Work out the finished part from the listing and answer in its coordinate system (mm). Face numbers are marked on the shaded views. A direction names the side the tool comes from. Coordinates: 2 decimals unless noted, no trailing zeros. Order: outer loops, then holes, each group sorted by start corner. A loop starts at its lowest first (then second) coordinate and runs counter-clockwise, first axis right, second up. Notation, with made-up numbers: M 81.5,-24.75 L 120.5,-24.75 A11 ccw 120.5,-12.75 Z; hole C 66,29.25 d7. An arc over 180 degrees is marked long. Write item = value, one per line. Start each with the question number.
Q1. Find section A-A on y = 25.5. Give the vertices of the cut face in (x, z).
Q2. Each of these flat-tipped pins is pushed along its axis until it touches: P1, Ø6.5, axis at x = 21, z = 0.5, coming from the +Y side; P2, Ø3, axis at x = 73, y = -20, coming from the +Z side; P3, Ø6.5, axis at y = 0.5, z = 0.5, coming from the -X side. Where does it stop, or does it pass through?
Q3. Determine the mould class of the marked faces 4, 5, 6 and 7 for opening direction Y: released by +Y, released by -Y, zero draft, split by the parting line, or undercut.
Q4. Find section B-B on z = 16. Give the vertices of the cut face in (x, y), and give its area (3 significant figures).
Q5. Find section C-C on y = -3.5. Give the vertices of the cut face in (x, z).
Q6. Straight lines are drawn through the part: line 1 along Z through (x, y) = (19.5, -15); line 2 along X through (y, z) = (12.5, 3); line 3 along X through (y, z) = (-12, 13). For each, find the intervals that lie inside material, in ascending order.
Q7. Find section D-D on z = 26. Give the vertices of the cut face in (x, y).
Q8. A tool of negligible diameter and unlimited length cuts with its end or side. For the marked faces 1, 2 and 3, from which of +Z, -Z, +X, -X, +Y, -Y can it reach the whole face along a straight path? Write none if from no direction.
```python
from build123d import *
from build123d import SkipClean  # not in build123d's __all__

# Parameters (mm, degrees)
F0_W          = 216.5604
F0_H          = 60.325
F1_DEPTH      = 11.176
F2_R          = 23.876
F2_R_2        = 12.7
F3_DEPTH      = 60.325
F5_DEPTH      = 60.326
F6_W          = 1.016
F6_H          = 60.325
F6_W_2        = 60.7332959771
F6_H_2        = 22.3266
F6_R          = 6.35
F7_DEPTH      = 22.353
F7_DEPTH_BACK = 23.877
F10_DEPTH     = 19.05
F11_DEPTH     = 19.05
F12_R         = 2.54
F13_R         = 7.874


# Not quite as in the source:
# - after a boolean that leaves OpenCascade's solid faulty, fix() repairs it


with BuildPart() as f1:
    # F0 (on Top) → F1 (new body, symmetric)
    with BuildSketch(Plane.XY):
        Rectangle(F0_W, F0_H)
    extrude(amount=F1_DEPTH, both=True)

    # F2 (on face) → F3 (join, through all)
    with BuildSketch(Plane.XZ.offset(30.1625)):
        with Locations((-85.9282, 11.176)):
            Circle(F2_R)
        with Locations((-85.9282, 11.176)):
            Circle(F2_R_2, mode=Mode.SUBTRACT)
    extrude(amount=-F3_DEPTH)

    # F4 (on face) → F5 (cut, through all)
    with BuildSketch(Plane.XZ.offset(30.1625)):
        with BuildLine():
            Line((-108.2802, -11.176), (-94.3217375141, -11.176))
            ThreePointArc((-94.3217375141, -11.176), (-102.8110815076, -5.7068815076), (-108.2802, 2.7824624859))
            Line((-108.2802, 2.7824624859), (-108.2802, -11.176))
        make_face()
        with BuildLine():
            Line((-77.5346624859, -11.176), (-94.3217375141, -11.176))
            ThreePointArc((-94.3217375141, -11.176), (-85.9282, -12.7), (-77.5346624859, -11.176))
        make_face()
        with BuildLine():
            ThreePointArc((-98.6282, 11.176), (-85.9282, -1.524), (-73.2282, 11.176))
            Line((-73.2282, 11.176), (-98.6282, 11.176))
        make_face()
    with SkipClean():  # cleaning this boolean's faces spoils the solid; the shape is the same uncleaned
        extrude(amount=-F5_DEPTH, mode=Mode.SUBTRACT)

    # F6 (on face) → F7 (cut, two sides)
    with BuildSketch(Plane.XY.offset(11.176)) as f7_sk:
        with Locations((107.7722, 0)):
            Rectangle(F6_W, F6_H)
        with Locations((-88.6705182493, 0)):
            Rectangle(F6_W_2, F6_H_2)
        with Locations((68.4022, -7.8105)):
            Circle(F6_R)
    with SkipClean():  # cleaning this boolean's faces spoils the solid; the shape is the same uncleaned
        extrude(amount=-F7_DEPTH, mode=Mode.SUBTRACT)
        extrude(f7_sk.sketch, amount=F7_DEPTH_BACK, mode=Mode.SUBTRACT)

    # F8 (on face) → F10 (cut)
    with BuildSketch(Plane(origin=(0, 30.1625, 0), x_dir=(-1, 0, 0), z_dir=(0, 1, 0))):
        Polygon((0.0762, 11.176), (-31.3182, 11.176), (-31.3182, -11.176), (-5.9182, -11.176), align=None)
    extrude(amount=-F10_DEPTH, mode=Mode.SUBTRACT)

    add(f1.part.fix(), mode=Mode.REPLACE)

    # F9 (on face) → F11 (join)
    with BuildSketch(Plane(origin=(0, 30.1625, 0), x_dir=(-1, 0, 0), z_dir=(0, 1, 0))):
        Polygon((-64.1604, 45.974), (-64.1604, -11.176), (-54.2544, -11.176), (-54.2544, 11.176), (-54.2544, 45.974), align=None)
        with BuildLine():
            Line((-54.2544, 45.974), (-54.2544, 11.176))
            Line((-54.2544, 11.176), (-31.3182, 11.176))
            ThreePointArc((-31.3182, 11.176), (-46.5191498234, 26.114588766), (-54.2544, 45.974))
        make_face()
    extrude(amount=-F11_DEPTH)

    add(f1.part.fix(), mode=Mode.REPLACE)

    # F12
    f12_edges = [f1.edges().sort_by_distance(p)[0] for p in [
        (-62.0522, 20.6629, 11.176),
        (-62.0522, -20.6629, 11.176),
        (64.1604, 20.6375, 45.974),
        (64.1604, 20.6375, 11.176),
    ]]
    fillet(f12_edges, radius=F12_R)

    # F13
    f13_edges = [f1.edges().sort_by_distance(p)[0] for p in [
        (107.2642, 0, 11.176),
    ]]
    fillet(f13_edges, radius=F13_R)


solid = f1.part
```
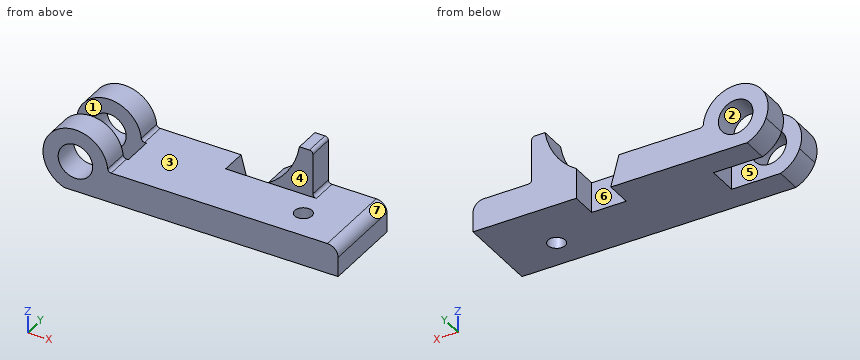
Findings below:
q1.outline = M -94.32,-11.18 L 5.92,-11.18 L -0.08,11.18 L -59.63,11.18 A2.54 cw -62.16,13.47 A23.88 ccw long Z; M 31.32,-11.18 L 107.26,-11.18 L 107.26,3.3 A7.87 ccw 99.39,11.18 L 66.7,11.18 A2.54 cw 64.16,13.72 L 64.16,43.43 A2.54 ccw 61.62,45.97 L 54.25,45.97 A50.8 cw 31.32,11.18 Z; hole C -85.93,11.18 d25.4
q2.P1 = 11.11
q2.P2 = 11.18
q2.P3 = -58.3
q3.face_4 = released by -Y
q3.face_5 = undercut
q3.face_6 = released by +Y
q3.face_7 = zero draft
q4.outline = M -109.31,-30.16 L -97.68,-30.16 L -97.68,-11.16 L -109.31,-11.16 Z; M -109.31,11.16 L -97.68,11.16 L -97.68,30.16 L -109.31,30.16 Z; M -74.18,-30.16 L -62.54,-30.16 L -62.54,-11.16 L -74.18,-11.16 Z; M -74.18,11.16 L -62.54,11.16 L -62.54,30.16 L -74.18,30.16 Z; M 37.74,11.11 L 64.16,11.11 L 64.16,30.16 L 37.74,30.16 Z
q4.area = 1,390 mm^2
q5.outline = M -58.3,-11.18 L 63.74,-11.18 L 63.74,11.18 L -58.3,11.18 Z; M 73.07,-11.18 L 107.26,-11.18 L 107.26,3.3 A7.87 ccw 99.39,11.18 L 73.07,11.18 Z
q6.line_1 = -11.18 to 11.18
q6.line_2 = -108.36 to -95.65, -76.21 to 2.12, 31.32 to 107.26
q6.line_3 = -109.73 to -98.5, -73.36 to -62.07
q7.outline = M -104.64,-30.16 L -67.21,-30.16 L -67.21,-11.16 L -104.64,-11.16 Z; M -104.64,11.16 L -67.21,11.16 L -67.21,30.16 L -104.64,30.16 Z; M 46.44,11.11 L 64.16,11.11 L 64.16,30.16 L 46.44,30.16 Z
q8.face_1 = +Z, -Z, -X
q8.face_2 = +Y, -Y
q8.face_3 = +Z, -Y
